The drawing under review shows one solid part. Ordinate dimensions are in mm from its lowest x, y, z. A direction names the side the tool comes from. Round coordinates to 2 decimals unless told otherwise and drop trailing zeros. Write each loop counter-clockwise with the first axis right and the second up, starting at its lowest first coordinate (ties: lowest second). Pieces come first, ordered by that corner, then holes. Notation, with made-up numbers: M 73,-10 L 114,-10 A7 cw 114,-5 Z; hole C 28,39.5 d2. An arc over 180 degrees is marked long. One line per item, written item: value. Start each with the question number.
1) Take a section at B-B, the plane z = 41.5. Write out the cut boundary in (x, y).
2) Take a section at C-C, the plane x = 83.5. Write out the cut boundary in (y, z), and give its area (3 significant figures).
3) Wall thickness on probe 1 along Z at (x, y) = (83, 43); probe 2 along X at (y, z) = (19.5, 58): over which ranges is each line inside the solid? List them lowest first.
4) For P1, Ø12.5, axis at y = 8.5, z = 62.5, coming from the +X side; P2, Ø4, axis at x = 76, y = 37, coming from the +Z side; P3, Ø1.5, axis at y = 27.5, z = 33, coming from the -X side, all flat-tipped, find the tip position at first contact; note any pin that passes through.
5) Tool access review of the marked faces 1, 2, 3 and 4: name each direction out of +Z, -Z, +X, -X, +Y, -Y from which nothing blocks a thin tool from reaching the whole face with its end or side.
6) Take a section at A-A, the plane y = 23. Write out the cut boundary in (x, z) (3 decimals).
7) Take a section at D-D, the plane y = 52.5. Write out the cut boundary in (x, z) (3 decimals).
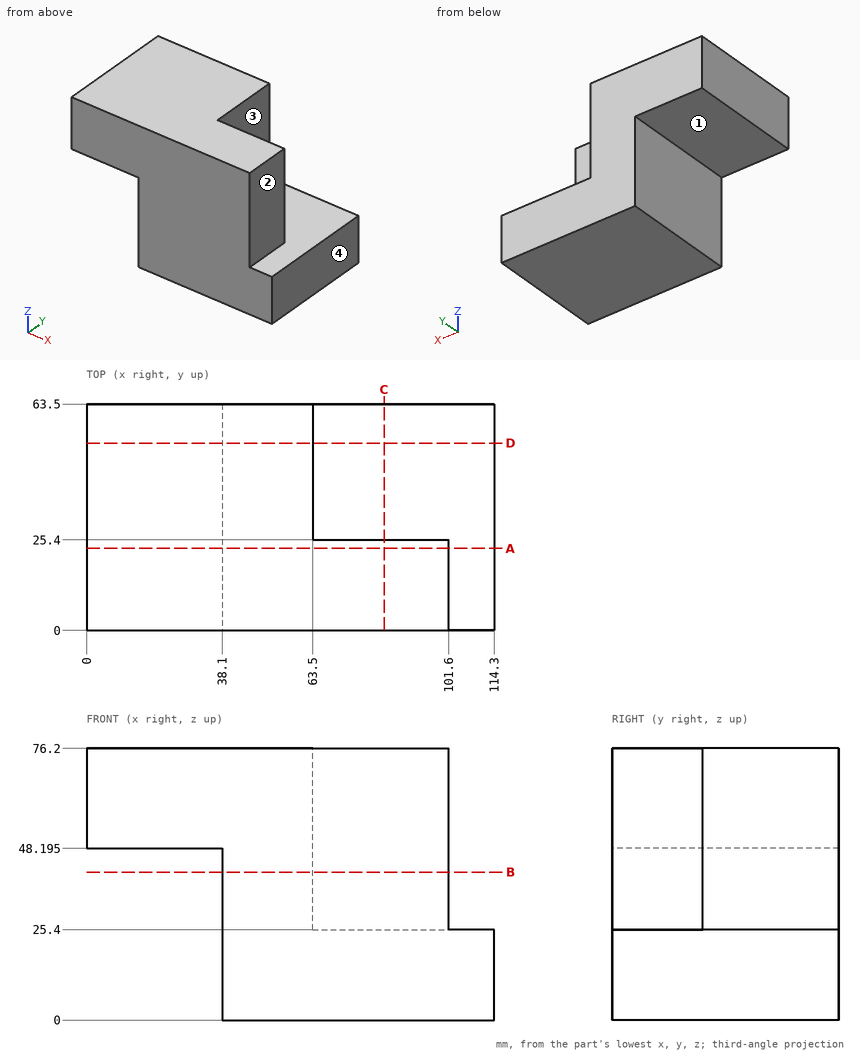
Checked values:
1. outline: M 38.1,0 L 101.6,0 L 101.6,25.4 L 63.5,25.4 L 63.5,63.5 L 38.1,63.5 Z
2. outline: M 0,0 L 63.5,0 L 63.5,25.4 L 25.4,25.4 L 25.4,76.2 L 0,76.2 Z
2. area: 2,900 mm2
3. probe 1: z = 0 to 25.4
3. probe 2: x = 0 to 101.6
4. P1: stops at x = 101.6
4. P2: stops at z = 25.4
4. P3: stops at x = 38.1
5. face 1: -Z, -X, +Y, -Y
5. face 2: +Z, +X, +Y, -Y
5. face 3: +Z, +X, +Y
5. face 4: +Z, -Z, +X, +Y, -Y
6. outline: M 0,48.195 L 38.1,48.195 L 38.1,0 L 114.3,0 L 114.3,25.4 L 101.6,25.4 L 101.6,76.2 L 0,76.2 Z
7. outline: M 0,48.195 L 38.1,48.195 L 38.1,0 L 114.3,0 L 114.3,25.4 L 63.5,25.4 L 63.5,76.2 L 0,76.2 Z
